Autodesk Inventor part; units mm, degrees
ref_plane "YZ Plane" through (0, 0, 0) normal (1, 0, 0) x (0, 1, 0)
ref_plane "XZ Plane" through (0, 0, 0) normal (0, 1, 0) x (-1, 0, 0)
ref_plane "XY Plane" through (0, 0, 0) normal (0, 0, 1) x (1, 0, 0)
sketch "Sketch1" plane through (0, 0, 0) normal (1, 0, 0) x (0, 1, 0)
  line L0 (0, 16) -> (4, 16) construction
  arc A0 (7.9892, 0) -> (4, 16) centre (-30.9916, -1.2217) ccw construction
  arc A1 (0, 12.5) -> (2.5, 15) centre (0, 15) ccw
  line L1 (0, 12.5) -> (0, 0) construction
  line L2 (4, 16) -> (2.5, 16)
  line L3 (2.5, 15) -> (2.5, 16)
  line L4 (7.9892, 0) -> (4, 0)
  line L5 (4, 10) -> (0, 10)
  line L6 (4, 10) -> (4, 0)
  line L7 (0, 12.5) -> (0, 10)
  line L8 (7.9892, 0) -> (4, 16)
  dimension "d0" = 4
  dimension "d3" = 5
  dimension "d4" = 1
  dimension "d5" = 4
  dimension "d11" = 10
  dimension "d12" = 16
  dimension "d13" = 104
revolve "Revolution1" add sketch "Sketch1" angle 360 about axis through (0, 0, 12.5) along (0, 0, -1)
sketch "Sketch2" plane through (0, 0, 0) normal (1, 0, 0) x (0, 1, 0)
  arc A0 (-2.5, 15) -> (2.5, 15) centre (0, 15) ccw
  circle A1 centre (0, 15) radius 1.5
  line L0 (0.6744, 16.3398) -> (-0.6744, 13.6602)
  point P0 (0, 0)
  dimension "d8" = 3
revolve "Revolution2" [suppressed]
properties part number "brush fitting"
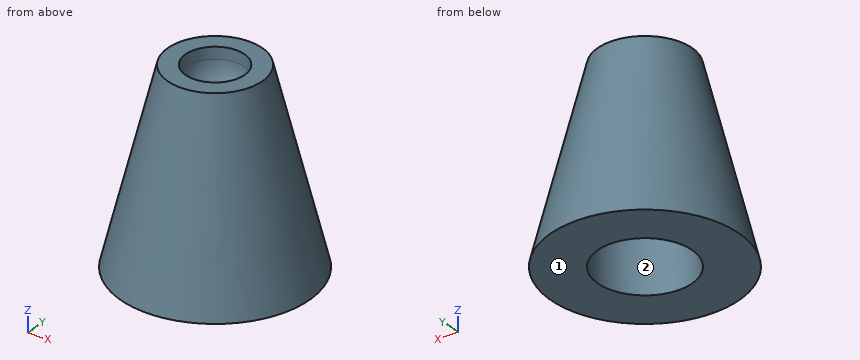
The listing builds one solid part. Answer for the finished solid, in the listing's coordinates (mm). Face numbers are marked on the shaded views. A direction names the side the tool comes from. Give positions to 0.01 mm unless a question says otherwise; leave off trailing zeros. Write each loop counter-clockwise with the first axis right and the second up, starting at its lowest first coordinate (ties: lowest second). Pieces come first, ordered by that corner, then holes. Notation, with made-up numbers: (30, -19) - (67, -19) arc R18 cw to (67, -7) - close; hole circle Ø5 at (-18, 10). An arc over 180 degrees is marked (long way). One line per question, with ' | ' between items. Start each with the question number.
1. Straight lines are drawn through the part: line 1 (X direction, y = 0, z = 6.75); line 2 (X direction, y = 0, z = 15.35); line 3 (Z direction, x = 1.25, y = 2.5). For each, find the intervals that lie inside material, in ascending order.
2. Section C-C, the plane z = 13 is taken. Determine the outline of the cut face in (x, y).
3. Given P1, Ø2, axis at y = 3, z = 5.5, coming from the +X side; P2, Ø3, axis at y = 5, z = 7.5, coming from the -X side; P3, Ø1, axis at y = -5, z = 5, coming from the -X side, each flat-ended and moving along its own axis, determine where each tip first touches the part or whether it passes through.
4. For the marked faces 1 and 2, determine the directions among +Z, -Z, +X, -X, +Y, -Y from which every point of the face is accessible in a straight line to the end or side of a thin tool.
5. Section D-D, the plane z = 3 is taken. Determine the outline of the cut face in (x, y), then the cut area to 3 significant figures.
6. Section A-A, the plane y = 0 is taken. Determine the outline of the cut face in (x, z).
Result:
1) line 1: x = -6.31 to -4, 4 to 6.31 | line 2: x = -4.16 to -2.5, 2.5 to 4.16 | line 3: z = 10 to 16
2) outline: circle Ø9.5 at (0, 0); hole circle Ø3 at (0, 0)
3) P1: stops at x = 6.4 | P2: stops at x = -5.11 | P3: stops at x = -5.05
4) face 1: -Z, +X, -X, +Y, -Y | face 2: -Z
5) outline: circle Ø14.48 at (0, 0); hole circle Ø8 at (0, 0) | area: 114 mm2
6) outline: (-7.99, 0) - (-4, 0) - (-4, 10) - (4, 10) - (4, 0) - (7.99, 0) - (4, 16) - (2.5, 16) - (2.5, 15) arc R2.5 cw to (-2.5, 15) - (-2.5, 16) - (-4, 16) - close
